Can you work these out from the model? Positions are in its coordinate system, mm. Round coordinates to 2 decimals unless told otherwise and drop trailing zeros. Order: outer loops, then holes, each group sorted by start corner. A loop starts at its lowest first (then second) coordinate and runs counter-clockwise, first axis right, second up.
Q1. We'd pull the mould along Y, two halves only. Please class faces 1 (the face through (-13, 14, 0)), 2 (the face through (-41.37, 28.21, 2.82)): pulls with the +Y half, pulls with the -Y half, needs draft (parallel to the pull), parting line crosses it, or undercut.
Q2. If we section it at A-A (y = -7.5): Please give me the cut outline in (x, z) (3 decimals), plus the area to 3 significant figures.
Q3. If we section it at D-D (y = 19.5): Please give me the cut outline in (x, z) (3 decimals), plus the area to 3 significant figures.
Q4. If I drill on line 1 (X direction, y = 5, z = 2.35); line 2 (X direction, y = -28, z = 4.55); line 3 (Y direction, x = -2, z = 3.55), over which ranges is the centre line in solid material (lowest first)?
Q5. If we section it at C-C (z = 1.25): Please give me the cut outline in (x, y), plus the area to 3 significant figures.
Q6. Will these pins go through, and if not, where does the flat tip stop? P1, Ø1, axis at y = 10.5, z = 2, coming from the -X side; P2, Ø3, axis at y = -24, z = 4.5, coming from the +X side.
Q7. If we section it at B-B (x = 15): Please give me the cut outline in (y, z) (3 decimals), plus the area to 3 significant figures.
from build123d import *

# Parameters (mm, degrees)
F1_DEPTH = 5.715


with BuildPart() as f1:
    # F0 (on Top) → F1 (new body)
    with BuildSketch(Plane.XY):
        with BuildLine():
            ThreePointArc((-12.466939, 11.319563), (-3.486683, 7.599819), (0.233061, -1.380437))
            Line((0.233061, -1.380437), (11.282061, -1.380437))
            ThreePointArc((11.282061, -1.380437), (16.587703, 27.674204), (-12.466939, 22.368563))
            Line((-12.466939, 22.368563), (-12.466939, 11.319563))
        make_face()
        with BuildLine():
            Line((11.282061, -1.380437), (0.233061, -1.380437))
            ThreePointArc((0.233061, -1.380437), (-3.486683, -10.360694), (-12.466939, -14.080437))
            Line((-12.466939, -14.080437), (-12.466939, -25.129437))
            ThreePointArc((-12.466939, -25.129437), (16.921955, -30.769331), (11.282061, -1.380437))
        make_face()
        with BuildLine():
            ThreePointArc((-25.166939, -1.380437), (-21.447195, 7.599819), (-12.466939, 11.319563))
            Line((-12.466939, 11.319563), (-12.466939, 22.368563))
            ThreePointArc((-12.466939, 22.368563), (-41.719379, 27.872003), (-36.215939, -1.380437))
            Line((-36.215939, -1.380437), (-25.166939, -1.380437))
        make_face()
        with BuildLine():
            Line((-12.466939, -25.129437), (-12.466939, -14.080437))
            ThreePointArc((-12.466939, -14.080437), (-21.447195, -10.360694), (-25.166939, -1.380437))
            Line((-25.166939, -1.380437), (-36.215939, -1.380437))
            ThreePointArc((-36.215939, -1.380437), (-41.964671, -30.87817), (-12.466939, -25.129437))
        make_face()
    extrude(amount=F1_DEPTH)


solid = f1.part
Solution:
1. face 1: needs draft
1. face 2: undercut
2. outline: (-43.872, 0) - (-23.595, 0) - (-23.595, 5.715) - (-43.872, 5.715) - close; (-1.339, 0) - (18.864, 0) - (18.864, 5.715) - (-1.339, 5.715) - close
2. area: 231 mm2
3. outline: (-46.46, 0) - (21.267, 0) - (21.267, 5.715) - (-46.46, 5.715) - close
3. area: 387 mm2
4. line 1: x = -43.89 to -23.45, -1.49 to 18.82
4. line 2: x = -44.31 to -14, -10.91 to 19.19
4. line 3: y = -34.99 to -8.57, 5.81 to 31.94
5. outline: (-36.22, -1.38) arc R18.12 ccw (long way) to (-12.47, -25.13) arc R18.08 ccw (long way) to (11.28, -1.38) arc R17.95 ccw (long way) to (-12.47, 22.37) arc R18.03 ccw (long way) to start; hole (-25.17, -1.38) arc R12.7 ccw to (-12.47, -14.08) arc R12.7 ccw to (0.23, -1.38) arc R12.7 ccw to start
5. area: 3,600 mm2
6. P1: stops at x = -46.52
6. P2: stops at x = 21.64
7. outline: (-32.438, 0) - (-3.536, 0) - (-3.536, 5.715) - (-32.438, 5.715) - close; (0.877, 0) - (29.084, 0) - (29.084, 5.715) - (0.877, 5.715) - close
7. area: 326 mm2
